Design review of the part built by this model. Coordinates are the model's own, in mm. Face numbers are marked on the shaded views. A direction names the side the tool comes from. Coordinates: 2 decimals unless noted, no trailing zeros. Loops run counter-clockwise (first coordinate to the right, second up) from the corner with the lowest first, then second, coordinate; pieces in that order, holes last. Notation, with made-up numbers: (-17, 45) -> (5, 45) arc R19 cw to (5, 70) -> close; hole circle Ø11 at (14, -24.75). An arc over 180 degrees is marked (long way). Use CSV: the item, a comma, the result in double quotes.
```python
from build123d import *

# Parameters (mm, degrees)
SKETCH1_W               = 20
SKETCH1_H               = 90
BOSS_EXTRUDE1_DEPTH     = 5
BOSS_EXTRUDE2_DEPTH     = 20
SKETCH3_W               = 50
SKETCH3_H               = 60
BOSS_EXTRUDE3_DEPTH     = 5
SKETCH6_W               = 20
SKETCH6_H               = 59.508572424
BOSS_EXTRUDE4_DEPTH     = 8
CUT_EXTRUDE3_DEPTH      = 10
CUT_EXTRUDE3_DEPTH_BACK = 20
SKETCH5_R               = 4
CUT_EXTRUDE4_DEPTH      = 20
SKETCH7_R               = 5
CUT_EXTRUDE5_DEPTH      = 2


with BuildPart() as part:
    # Sketch1 → Boss-Extrude1 (new body)
    with BuildSketch(Plane(origin=(0, 0, 0), x_dir=(1, 0, 0), z_dir=(0, 1, 0))):
        Rectangle(SKETCH1_W, SKETCH1_H)
    extrude(amount=BOSS_EXTRUDE1_DEPTH)

    # Sketch2 → Boss-Extrude2 (add)
    with BuildSketch(Plane(origin=(10, 0, 0), x_dir=(0, 0, -1), z_dir=(1, 0, 0))):
        Polygon((-45, 0), (-29.672384363, -9.999664599), (0.081901849, -9.999664599), (0, 0), align=None)
        Polygon((0, 0), (0.081901849, -9.999664599), (29.836188061, -9.999664599), (45, 0), align=None)
    extrude(amount=-BOSS_EXTRUDE2_DEPTH)

    # Sketch6 → Boss-Extrude4 (add)
    with BuildSketch(Plane.XZ.offset(9.999664599)):
        with Locations((0, -0.081901849)):
            Rectangle(SKETCH6_W, SKETCH6_H)
    extrude(amount=BOSS_EXTRUDE4_DEPTH)


with BuildPart() as body_2:
    # Sketch3 → Boss-Extrude3 (new body)
    with BuildSketch(Plane(origin=(0, -28.999664599, 0), x_dir=(-1, 0, 0), z_dir=(0, -1, 0))):
        Rectangle(SKETCH3_W, SKETCH3_H)
    extrude(amount=BOSS_EXTRUDE3_DEPTH)


    add(part.part)  # loft3 joins it to this body
    # loft from a face of the part (loft3)
    loft([body_2.faces().sort_by_distance((0, -28.999664599, 0))[0], body_2.faces().sort_by_distance((0, -17.999664599, -0.081901849))[0]])

    # Sketch4 → Cut-Extrude3 (cut, two sides: drawn at the far end of the back side and taken through both)
    with BuildSketch(Plane.XZ.offset(33.999664599).offset(-CUT_EXTRUDE3_DEPTH_BACK)):
        with BuildLine():
            ThreePointArc((-13.080007345, 22), (-14.251580221, 24.828427125), (-17.080007345, 26))
            Line((-17.080007345, 26), (-17.080007345, 22))
            Line((-17.080007345, 22), (-21.080007345, 22))
            ThreePointArc((-21.080007345, 22), (-17.080007345, 18), (-13.080007345, 22))
        make_face()
        with BuildLine():
            Line((-17.080007345, 22), (-17.080007345, 26))
            ThreePointArc((-17.080007345, 26), (-19.90843447, 24.828427125), (-21.080007345, 22))
            Line((-21.080007345, 22), (-17.080007345, 22))
        make_face()
        with BuildLine():
            ThreePointArc((21, 22), (19.828427125, 24.828427125), (17, 26))
            Line((17, 26), (17, 22))
            Line((17, 22), (21, 22))
        make_face()
        with BuildLine():
            Line((17, 22), (17, 26))
            ThreePointArc((17, 26), (14.171572875, 19.171572875), (21, 22))
            Line((21, 22), (17, 22))
        make_face()
        with BuildLine():
            ThreePointArc((-21, -22), (-19.828427125, -24.828427125), (-17, -26))
            Line((-17, -26), (-17, -22))
            Line((-17, -22), (-21, -22))
        make_face()
        with BuildLine():
            Line((-17, -22), (-17, -26))
            ThreePointArc((-17, -26), (-14.171572875, -24.828427125), (-13, -22))
            ThreePointArc((-13, -22), (-17, -18), (-21, -22))
            Line((-21, -22), (-17, -22))
        make_face()
        with BuildLine():
            ThreePointArc((21, -22), (14.171572875, -19.171572875), (17, -26))
            Line((17, -26), (17, -22))
            Line((17, -22), (21, -22))
        make_face()
        with BuildLine():
            Line((17, -22), (17, -26))
            ThreePointArc((17, -26), (19.828427125, -24.828427125), (21, -22))
            Line((21, -22), (17, -22))
        make_face()
    extrude(amount=CUT_EXTRUDE3_DEPTH + CUT_EXTRUDE3_DEPTH_BACK, mode=Mode.SUBTRACT)

    # Sketch5 → Cut-Extrude4 (cut)
    with BuildSketch(Plane(origin=(0, 5, 0), x_dir=(1, 0, 0), z_dir=(0, 1, 0))):
        with Locations(Location((0, 38, 0), (0, 0, 270))):
            Circle(SKETCH5_R)
        with Locations(Location((0, -38, 0), (0, 0, 270))):
            Circle(SKETCH5_R)
    extrude(amount=-CUT_EXTRUDE4_DEPTH, mode=Mode.SUBTRACT)

    # Sketch7 → Cut-Extrude5 (cut)
    with BuildSketch(Plane.XZ.offset(33.999664599)):
        with Locations(Location((0, 0, 0), (0, 0, 270))):
            Circle(SKETCH7_R)
    extrude(amount=-CUT_EXTRUDE5_DEPTH, mode=Mode.SUBTRACT)


solid = body_2.part
```
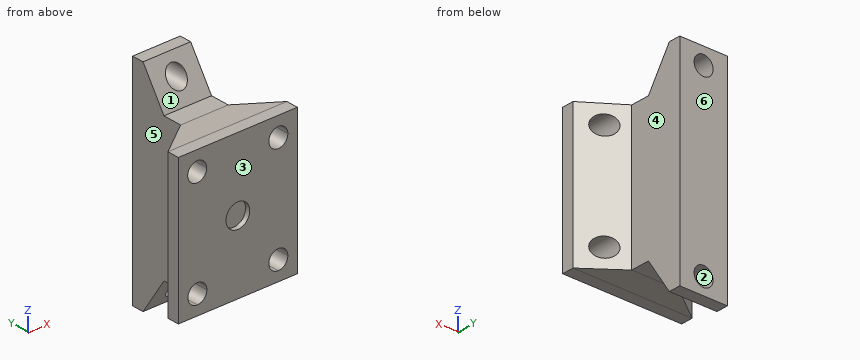
Item 1: Add section B-B (z = -37). Give the boundary of the cut face in (x, y).
Checked values:
outline,"(-10, -5.28) -> (-3.87, -5.28) -> (-3.87, 5) -> (-10, 5) -> close; (3.87, -5.28) -> (10, -5.28) -> (10, 5) -> (3.87, 5) -> close"
Item 2: Draft analysis for pull direction Z (two halves, no side actions). For the marked faces 1, 2 and 3, state which applies: pulls with the +Z half, pulls with the -Z half, needs draft (parallel to the pull), parting line crosses it, or undercut.
Checked values:
face 1,"pulls with the +Z half"
face 2,"undercut"
face 3,"needs draft"
Item 3: Clearance check with flat-ended pins moving along their axes: pin 1 (5 mm diameter, centred on x = 10.5, y = -22.5, fed in from +Z); pin 2 (6.5 mm diameter, centred on x = 4, y = -15.5, fed in from +Z); pin 3 (4 mm diameter, centred on x = 9.5, y = -30.5, fed in from -Z); pin 4 (11 mm diameter, centred on x = 1, z = -2, fed in from -Y). State where each tip first meets the part, or that it passes through.
Checked values:
pin 1,"z = 29.88"
pin 2,"z = 29.69"
pin 3,"z = -30"
pin 4,"y = -34"
Item 4: Machinability: for the marked faces 4, 5 and 6, which of the approach directions +Z, -Z, +X, -X, +Y, -Y give a long, thin tool a straight path to every point of the face, cutting with its end or side? Answer none if there is none.
Checked values:
face 4,"+Z, -Z, +X, +Y"
face 5,"+Z, -Z, -X, +Y"
face 6,"+Z, -Z, +X, -X, +Y"
Item 5: Add section C-C (x = 0). State how many separate pieces and enclosed holes the cut face has, then the cut area to 3 significant figures.
Checked values:
separate pieces,"3"
enclosed holes,"0"
area,"2,460 mm^2"
Item 6: To check wall thickness, follow line 1 along Z through (x, y) = (17, -29.75); line 2 along Z through (x, y) = (0, 0); line 3 along X through (y, z) = (-27, 20.5). State the ranges of each line that lie inside material, in increasing order.
Checked values:
line 1,"-30 to -26, -18 to 18, 26 to 30"
line 2,"-45 to -42, -34 to 34, 42 to 45"
line 3,"-22.27 to -20.79, -13.37 to 13.29, 20.71 to 22.27"
Item 7: Add section A-A (y = -3.5). Give the boundary of the cut face in (x, z).
Checked values:
outline,"(-10, -39.69) -> (-3.62, -39.69) arc R4 cw (long way) to (3.62, -39.69) -> (10, -39.69) -> (10, 39.64) -> (3.65, 39.64) arc R4 cw (long way) to (-3.65, 39.64) -> (-10, 39.64) -> close"
